Job drawing, mm, ordinate dimensions from the low corner. One solid piece. Round coordinates to 2 decimals unless told otherwise and drop trailing zeros. Loops run counter-clockwise (first coordinate to the right, second up) from the corner with the lowest first, then second, coordinate; pieces in that order, holes last.
1) Drop flat-ended pins along their axis: P1, Ø5, axis at x = 6.477, z = 22.479, coming from the +Y side (3 decimals); P2, Ø2, axis at x = 6.477, z = 2.921, coming from the -Y side. Give the stop position or say it passes through.
2) Band-saw the part on B-B, the plane z = 2. Write the cut outline in (x, y) (1 decimal).
3) Probe line 1 (Z direction, x = 89, y = 1.1) (1 decimal); line 2 (Z direction, x = 88.5, y = 0.45) (1 decimal); line 3 (X direction, y = 1.9, z = 6.5) (1 decimal). List the from-to ranges inside material, lowest first.
4) Band-saw the part on A-A, the plane y = 1.5. State how many separate pieces and enclosed holes the cut face has, then the cut area to 3 significant figures.
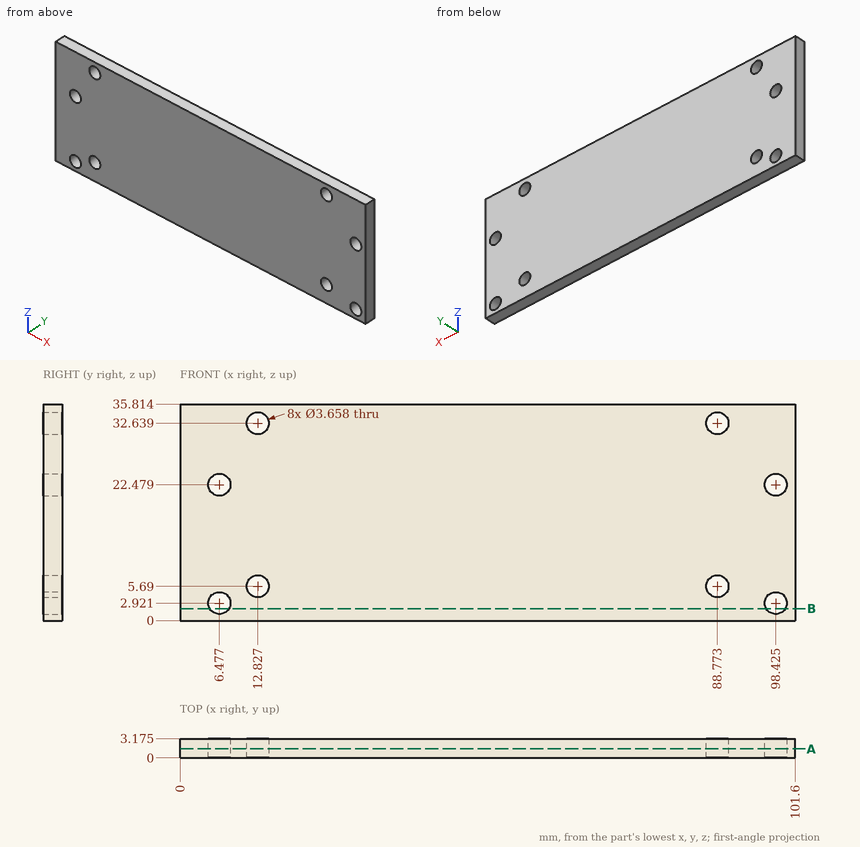
Reported:
1. P1: stops at y = 3.175
1. P2: passes through
2. outline: (0, 0) - (4.9, 0) - (4.9, 3.2) - (0, 3.2) - close; (8.1, 0) - (96.8, 0) - (96.8, 3.2) - (8.1, 3.2) - close; (100, 0) - (101.6, 0) - (101.6, 3.2) - (100, 3.2) - close
3. line 1: z = 0 to 3.9, 7.5 to 30.8, 34.5 to 35.8
3. line 2: z = 0 to 3.9, 7.5 to 30.8, 34.4 to 35.8
3. line 3: x = 0 to 11.2, 14.5 to 87.1, 90.4 to 101.6
4. separate pieces: 1
4. enclosed holes: 8
4. area: 3,550 mm2
